Build history of the part. All positions in model axes, mm. Face numbers are marked on the shaded views. A direction names the side the tool comes from. Coordinates: 2 decimals unless noted, no trailing zeros. Write each loop counter-clockwise with the first axis right and the second up, starting at its lowest first coordinate (ties: lowest second). Pieces come first, ordered by that corner, then holes.
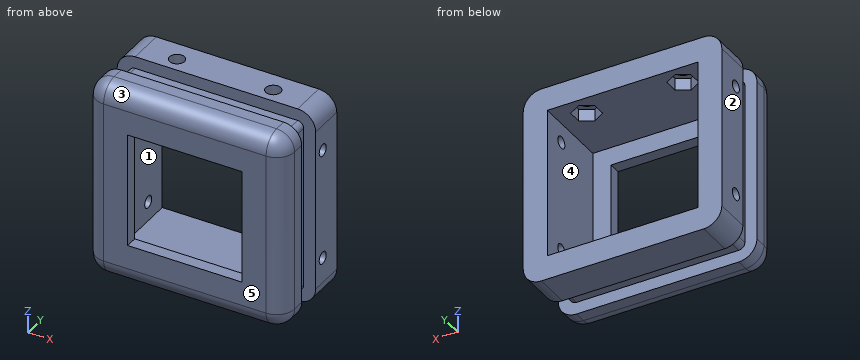
```python
from build123d import *

# Parameters (mm, degrees)
SKETCH_1_W          = 33
SKETCH_1_H          = 33
SKETCH_1_W_2        = 13
SKETCH_1_H_2        = 13
EXTRUDE_1_DEPTH     = 15
SKETCH_2_W          = 25
SKETCH_2_H          = 25
CUT_EXTRUDE_1_DEPTH = 13
FILLET_3_R          = 3
SKETCH_4_R          = 1
CUT_EXTRUDE_2_DEPTH = 43.930175867
SKETCH_11_W         = 19
SKETCH_11_H         = 19
CUT_EXTRUDE_5_DEPTH = 2
SKETCH_14_W         = 4
SKETCH_14_H         = 2
CUT_EXTRUDE_6_DEPTH = 2
SKETCH_20_R         = 1.25
CUT_EXTRUDE_7_DEPTH = 42.412558482


with BuildPart() as part:
    # Эскиз1 → Бобышка-Вытянуть1 (new body)
    with BuildSketch(Plane(origin=(0, 0, 0), x_dir=(1, 0, 0), z_dir=(0, 1, 0))):
        with Locations((6.5, 6.5)):
            Rectangle(SKETCH_1_W, SKETCH_1_H)
        with Locations((6.5, 6.5)):
            Rectangle(SKETCH_1_W_2, SKETCH_1_H_2, mode=Mode.SUBTRACT)
    extrude(amount=EXTRUDE_1_DEPTH)

    # Эскиз2 → Вырез-Вытянуть1 (cut)
    with BuildSketch(Plane(origin=(0, 15, 0), x_dir=(1, 0, 0), z_dir=(0, 1, 0))):
        with Locations((6.5, 6.5)):
            Rectangle(SKETCH_2_W, SKETCH_2_H)
    extrude(amount=-CUT_EXTRUDE_1_DEPTH, mode=Mode.SUBTRACT)

    # Скругление3
    fillet_3_edges = [part.edges().sort_by_distance(p)[0] for p in [
        (6.5, 0, -23),
        (23, 0, -6.5),
        (6.5, 0, 10),
        (-10, 0, -6.5),
        (-10, 7.5, -23),
        (23, 7.5, -23),
        (23, 7.5, 10),
        (-10, 7.5, 10),
    ]]
    fillet(fillet_3_edges, radius=FILLET_3_R)

    # Эскиз4 → Вырез-Вытянуть2 (cut, through all)
    with BuildSketch(Plane.ZY.offset(10)):
        with Locations((2.75, 11)):
            Circle(SKETCH_4_R)
        with Locations((-15.75, 11)):
            Circle(SKETCH_4_R)
    extrude(amount=-CUT_EXTRUDE_2_DEPTH, mode=Mode.SUBTRACT)

    # Эскиз11 → Вырез-Вытянуть5 (cut)
    with BuildSketch(Plane.XZ):
        with Locations((6.5, -6.5)):
            Rectangle(SKETCH_11_W, SKETCH_11_H)
    extrude(amount=-CUT_EXTRUDE_5_DEPTH, mode=Mode.SUBTRACT)

    # Вырез-По траектории2: sweep along a path in Эскиз16
    with BuildLine(Plane(origin=(0, 7, 0), x_dir=(0, 0, 1), z_dir=(0, -1, 0))) as sweep_2_path:
        Line((-23, 7), (-23, -20))
        ThreePointArc((-23, -20), (-22.121320344, -22.121320344), (-20, -23))
        Line((-20, -23), (7, -23))
        ThreePointArc((7, -23), (9.121320344, -22.121320344), (10, -20))
        Line((10, -20), (10, 7))
        ThreePointArc((10, 7), (9.121320344, 9.121320344), (7, 10))
        Line((7, 10), (-20, 10))
        ThreePointArc((-20, 10), (-22.121320344, 9.121320344), (-23, 7))
    # Эскиз14 → Вырез-По траектории2 (sweep, cut)
    with BuildSketch(Plane(origin=(-7, 0, 0), x_dir=(0, 1, 0), z_dir=(-1, 0, 0))):
        with Locations((7, 22)):
            Rectangle(SKETCH_14_W, SKETCH_14_H)
    sweep(path=sweep_2_path.line, mode=Mode.SUBTRACT)

    # Эскиз18 → Вырез-Вытянуть6 (cut)
    with BuildSketch(Plane(origin=(0, 0, 6), x_dir=(-1, 0, 0), z_dir=(0, 0, -1))):
        Polygon((-0.5, 10.345299462), (1.5, 9.190598923), (3.5, 10.345299462), (3.5, 12.654700538), (1.5, 13.809401077), (-0.5, 12.654700538), align=None)
        Polygon((-16.5, 10.345299462), (-14.5, 9.190598923), (-12.5, 10.345299462), (-12.5, 12.654700538), (-14.5, 13.809401077), (-16.5, 12.654700538), align=None)
    extrude(amount=-CUT_EXTRUDE_6_DEPTH, mode=Mode.SUBTRACT)

    # Эскиз20 → Вырез-Вытянуть7 (cut, through all)
    with BuildSketch(Plane(origin=(0, 0, 8), x_dir=(-1, 0, 0), z_dir=(0, 0, -1))):
        with Locations((-14.5, 11.5)):
            Circle(SKETCH_20_R)
        with Locations((1.5, 11.5)):
            Circle(SKETCH_20_R)
    extrude(amount=-CUT_EXTRUDE_7_DEPTH, mode=Mode.SUBTRACT)


solid = part.part
```
1. Saw through at B-B on x = 15. State how many separate pieces and enclosed holes the cut face has, plus the area to 3 significant figures.
Computed values:
separate pieces: 3
enclosed holes: 0
area: 99.5 mm2
2. 3-axis set-ups, long thin cutter, end or side, ignore diameter. For the marked faces 1 and 2: which of +Z, -Z, +X, -X, +Y, -Y reach the whole face in a straight line?
Computed values:
face 1: +Y
face 2: +Z, -Z, -X, +Y, -Y
3. Saw through at C-C on y = 1.25. List the corners of the cut face in (x, z), plus the area to 3 significant figures.
Computed values:
outline: (-9.44, -20) arc R2.44 ccw to (-7, -22.44) - (20, -22.44) arc R2.44 ccw to (22.44, -20) - (22.44, 7) arc R2.44 ccw to (20, 9.44) - (-7, 9.44) arc R2.44 ccw to (-9.44, 7) - close; hole (-3, -16) - (16, -16) - (16, 3) - (-3, 3) - close
area: 650 mm2
4. Mould opens along Z. For the marked faces 3, 4 and 5 say: +Z half, -Z half, draft (parallel to the pull), parting line (faces both ways), or undercut.
Computed values:
face 3: +Z half
face 4: undercut
face 5: draft
5. Probe line 1 along Y through (x, z) = (-8.65, -15.75); line 2 along X through (y, z) = (9.75, -17.5); line 3 along Y through (x, z) = (19.95, 2.75). List the from-to ranges inside material, lowest first.
Computed values:
line 1: y = 0.49 to 5, 9 to 10, 12 to 15
line 2: x = -10 to -6, 19 to 23
line 3: y = 0 to 10, 12 to 15
6. Flat gauge pins, fed straight in: pin 1 (3 mm diameter, centred on y = 7, z = -4.5, fed in from -X); pin 2 (1.2 mm diameter, centred on y = 7.5, z = -3.5, fed in from +X); pin 3 (6 mm diameter, centred on x = 14, z = -2, fed in from +Y). Where does each tip first touch, or does it go through?
Computed values:
pin 1: stops at x = -8
pin 2: stops at x = 21
pin 3: stops at y = 2
7. Saw through at A-A on z = -5.5. List the corners of the cut face in (x, y), plus the area to 3 significant figures.
Computed values:
outline: (-10, 3) arc R3 ccw to (-7, 0) - (-3, 0) - (-3, 2) - (-6, 2) - (-6, 15) - (-10, 15) - (-10, 9) - (-8, 9) - (-8, 5) - (-10, 5) - close; (16, 0) - (20, 0) arc R3 ccw to (23, 3) - (23, 5) - (21, 5) - (21, 9) - (23, 9) - (23, 15) - (19, 15) - (19, 2) - (16, 2) - close
area: 112 mm2
